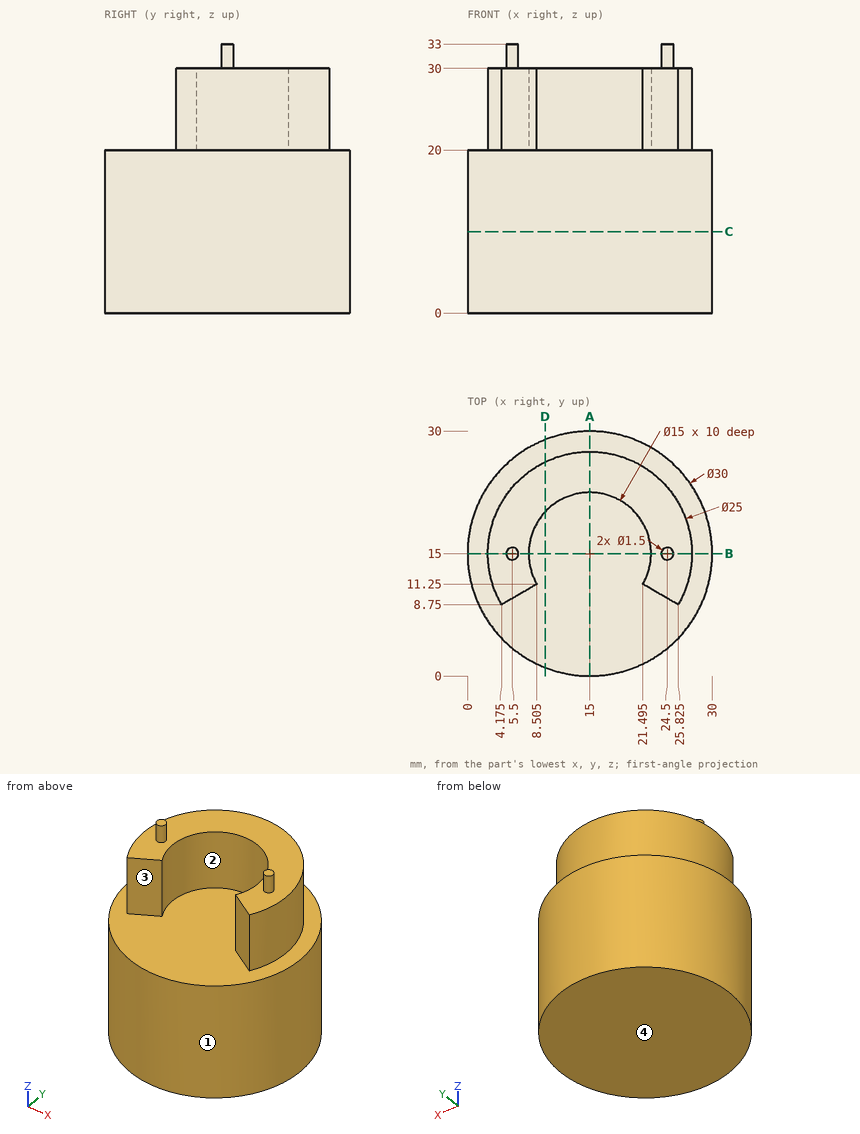
Verification items for this drawing (mm, ordinates from the low corner). Round coordinates to 2 decimals unless told otherwise and drop trailing zeros. Order: outer loops, then holes, each group sorted by start corner. A loop starts at its lowest first (then second) coordinate and runs counter-clockwise, first axis right, second up. Notation, with made-up numbers: (72, 84.5) - (103, 84.5) arc R30 ccw to (103, 123.5) - close; hole circle Ø10 at (24.25, 37.5). An arc over 180 degrees is marked (long way). Use CSV: the item, a comma, the result in double quotes.
(1) Section check C-C on z = 10. Record the boundary of the cut face in (x, y), and give its area (3 significant figures).
Entries:
outline,"circle Ø30 at (15, 15)"
area,"707 mm^2"
(2) Thickness scan on probe 1 along X at (y, z) = (15, 24.5); probe 2 along Z at (x, y) = (28.5, 10.75); probe 3 along Z at (x, y) = (7.75, 18). Record the ranges inside material, lowest first. Write a range as from..to.
Entries:
probe 1,"2.5..7.5, 22.5..27.5"
probe 2,"0..20"
probe 3,"0..30"
(3) Mould release check, pull along Y, two halves, no side actions. Record for the marked faces 1, 2, 3 and 4: released by +Y, released by -Y, zero draft, split by the parting line, or undercut.
Entries:
face 1,"split by the parting line"
face 2,"undercut"
face 3,"released by -Y"
face 4,"zero draft"
(4) Section check D-D on x = 9.5. Record the boundary of the cut face in (y, z) (1 decimal).
Entries:
outline,"(1, 0) - (29, 0) - (29, 20) - (26.2, 20) - (26.2, 30) - (20.1, 30) - (20.1, 20) - (1, 20) - close"
(5) Gauge pin test, flat ends, axial feed: pin 1 Ø1 at (x, y) = (8, 18.5) entering from +Z; pin 2 Ø6 at (y, z) = (24, 10) entering from -X; pin 3 Ø12 at (x, z) = (4, 27.5) entering from -Y. Record the tip position at first contact, or that the pin passes through.
Entries:
pin 1,"z = 30"
pin 2,"x = 1.25"
pin 3,"y = 8.75"
(6) Section check A-A on x = 15. Record the boundary of the cut face in (y, z), and give its area (3 significant figures).
Entries:
outline,"(0, 0) - (30, 0) - (30, 20) - (27.5, 20) - (27.5, 30) - (22.5, 30) - (22.5, 20) - (0, 20) - close"
area,"650 mm^2"
(7) Section check B-B on y = 15. Record the boundary of the cut face in (x, z).
Entries:
outline,"(0, 0) - (30, 0) - (30, 20) - (27.5, 20) - (27.5, 30) - (25.25, 30) - (25.25, 33) - (23.75, 33) - (23.75, 30) - (22.5, 30) - (22.5, 20) - (7.5, 20) - (7.5, 30) - (6.25, 30) - (6.25, 33) - (4.75, 33) - (4.75, 30) - (2.5, 30) - (2.5, 20) - (0, 20) - close"
